Drawing for the job (mm, zero at the part's lowest x, y, z). Round coordinates to 2 decimals unless told otherwise and drop trailing zeros. Loops run counter-clockwise (first coordinate to the right, second up) from the corner with the lowest first, then second, coordinate; pieces in that order, holes last. Notation, with made-up numbers: M 17,11.5 L 51,11.5 A10 ccw 51,18.5 Z; hole C -16,15 d5. An arc over 180 degrees is marked long. Use a Markdown table: item, result. Add a question column.
Q1. Cut at A-A (x = 141). Give the cut face in (y, z).
Q2. Probe line 1 (Y direction, x = 16, z = 47.2). List the from-to ranges inside material, lowest first. Write a range as from..to.
Q3. Pin check, flat tip, straight feed: pin 1 (13 mm diameter, centred on x = 16, y = 17.5, fed in from +Z). Stop position of the tip, or through.
Q4. Mould opens along X. For the marked faces 1, 2, 3 and 4 say: +X half, -X half, draft (parallel to the pull), parting line (faces both ways), or undercut.
Q5. Cut at B-B (x = 15). Give the cut face in (y, z).
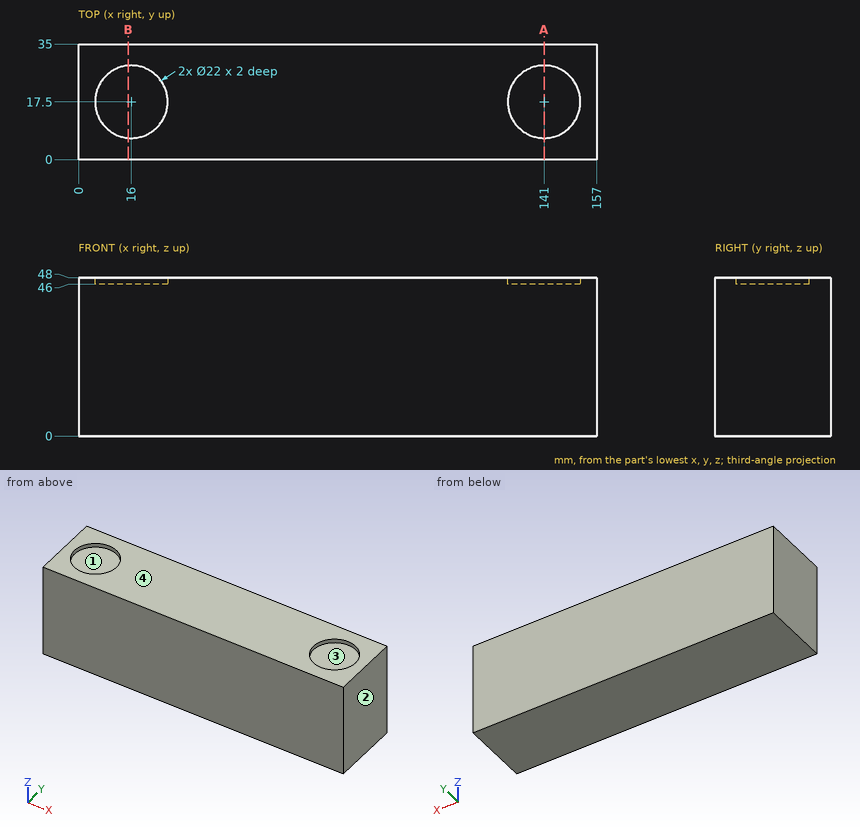
Checked values:
| question | item | result |
|---|---|---|
| 1 | outline | M 0,0 L 35,0 L 35,48 L 28.5,48 L 28.5,46 L 6.5,46 L 6.5,48 L 0,48 Z |
| 2 | line 1 | y = 0..6.5, 28.5..35 |
| 3 | pin 1 | stops at z = 46 |
| 4 | face 1 | undercut |
| 4 | face 2 | +X half |
| 4 | face 3 | undercut |
| 4 | face 4 | draft |
| 5 | outline | M 0,0 L 35,0 L 35,48 L 28.45,48 L 28.45,46 L 6.55,46 L 6.55,48 L 0,48 Z |
